Could you check a few things on this drawing? It's one solid part, dimensions in mm from its lowest x, y, z. A direction names the side the tool comes from. Give positions to 0.01 mm unless a question says otherwise; leave off trailing zeros. Loops run counter-clockwise (first coordinate to the right, second up) from the corner with the lowest first, then second, coordinate; pieces in that order, holes last. Notation, with made-up numbers: (74.5, -15.75) - (116.5, -15.75) arc R23 cw to (116.5, -3.75) - close; hole circle Ø10 at (-1.5, 52). An arc over 180 degrees is marked (long way). Write item = value, one per line.
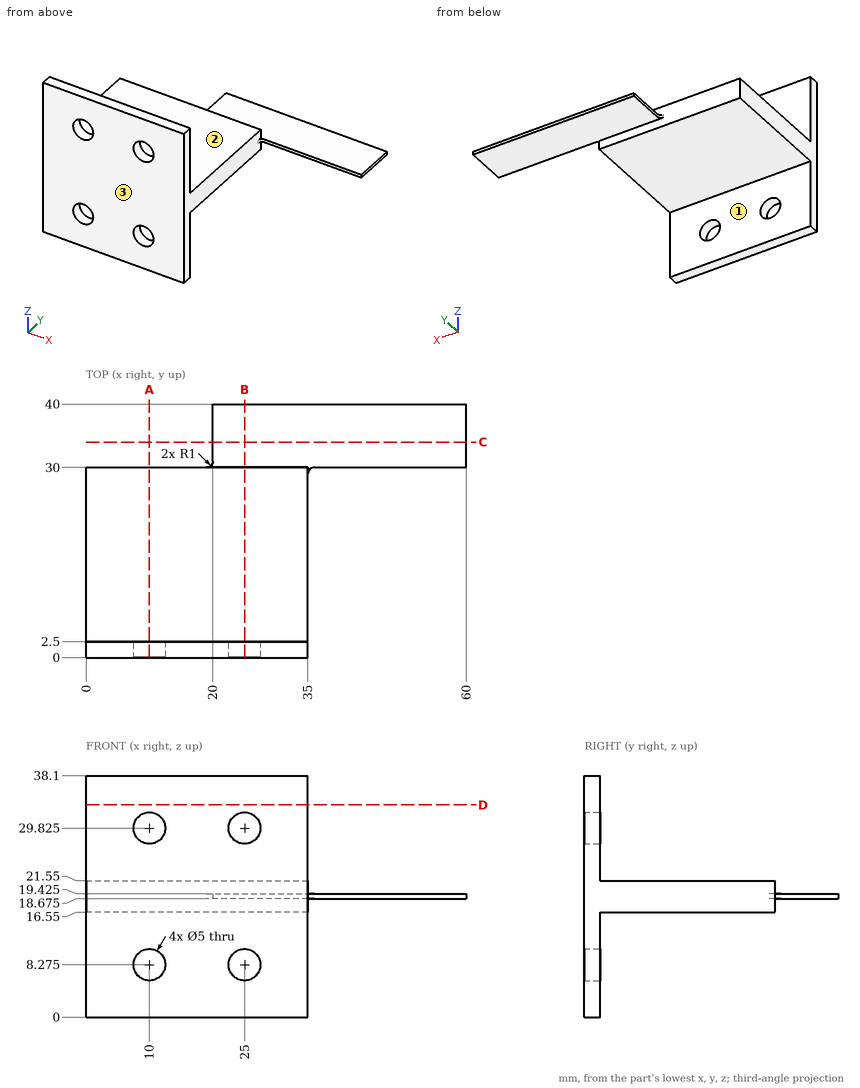
Q1. Imagine slicing it at C-C, the plane y = 34. Write out the boundary of the cut face in (x, z) (3 decimals), then the cut area to 3 significant figures.
Output:
outline = (20, 18.675) - (60, 18.675) - (60, 19.425) - (20, 19.425) - close
area = 30.0 mm2
Q2. For pin 1 (10 mm diameter, centred on x = 41, y = 10.5, fed in from -Z); pin 2 (6.5 mm diameter, centred on x = 25, z = 8.275, fed in from +Y); pin 3 (6 mm diameter, centred on y = 13.5, z = 21.5, fed in from +X); pin 4 (0.6 mm diameter, centred on x = 45.5, z = 19, fed in from -Y), each with a flat end and sliding along its axis, tell me the tip position at first contact or that it passes through.
Output:
pin_1 = through
pin_2 = 2.5
pin_3 = 35
pin_4 = 30
Q3. Imagine slicing it at B-B, the plane x = 25. Write out the boundary of the cut face in (y, z) (3 decimals), then the cut area to 3 significant figures.
Output:
outline = (0, 0) - (2.5, 0) - (2.5, 5.775) - (0, 5.775) - close; (0, 10.775) - (2.5, 10.775) - (2.5, 16.55) - (30, 16.55) - (30, 18.675) - (40, 18.675) - (40, 19.425) - (30, 19.425) - (30, 21.55) - (2.5, 21.55) - (2.5, 27.325) - (0, 27.325) - close; (0, 32.325) - (2.5, 32.325) - (2.5, 38.1) - (0, 38.1) - close
area = 215 mm2
Q4. Imagine slicing it at A-A, the plane x = 10. Write out the boundary of the cut face in (y, z) (3 decimals).
Output:
outline = (0, 0) - (2.5, 0) - (2.5, 5.775) - (0, 5.775) - close; (0, 10.775) - (2.5, 10.775) - (2.5, 16.55) - (30, 16.55) - (30, 21.55) - (2.5, 21.55) - (2.5, 27.325) - (0, 27.325) - close; (0, 32.325) - (2.5, 32.325) - (2.5, 38.1) - (0, 38.1) - close
Q5. Imagine slicing it at D-D, the plane z = 33.5. Write out the boundary of the cut face in (x, y), then the cut area to 3 significant figures.
Output:
outline = (0, 0) - (35, 0) - (35, 2.5) - (0, 2.5) - close
area = 87.5 mm2
Q6. I need wall thicknesses on L1, parallel to Z at x = 10, y = 0.5 (3 decimals); L2, parallel to Z at x = 19.5, y = 6.5; L3, parallel to Y at x = 34.5, z = 30. Which ranges of each line are inside material? Lowest first, please.
Output:
L1 = 0 to 5.775, 10.775 to 27.325, 32.325 to 38.1
L2 = 16.55 to 21.55
L3 = 0 to 2.5
Q7. Which directions (+Z, -Z, +X, -X, +Y, -Y) give clear straight access to the entire face, cutting with the end or side of a thin tool? Please do the marked faces 1, 2 and 3.
Output:
face_1 = -Z, +X, -X, +Y
face_2 = +Z, +X, -X, +Y
face_3 = +Z, -Z, +X, -X, -Y
